Can you work these out from the model? Positions are in its coordinate system, mm. Face numbers are marked on the shaded views. Give positions to 0.01 mm unless a question says otherwise; leave off trailing zeros. Write each loop counter-clockwise with the first axis right and the second up, starting at its lowest first coordinate (ties: lowest second). Pieces come first, ordered by that corner, then holes. Notation, with made-up numbers: (-28, -14) -> (-12, -14) arc R5 ccw to (-12, -6) -> close; hole circle Ø11 at (-12, -0.5). An arc over 180 degrees is marked (long way). Answer as CSV lines item,"result". Start each with the question number.
1. I need wall thicknesses on line 1 (X direction, y = -26, z = 5); line 2 (Y direction, x = -15.5, z = 3.5); line 3 (X direction, y = -1, z = 5). Which ranges of each line are inside material? Lowest first, please. Write a range as [from, to].
2. If we section it at A-A on y = -14.5: Write out the boundary of the cut face in (x, z), plus the area to 3 significant figures.
3. If we section it at B-B on z = 2.25: Write out the boundary of the cut face in (x, y).
4. If we section it at C-C on y = 40.5: Write out the boundary of the cut face in (x, z), plus the area to 3 significant figures.
5. If we mould it in two halves opening along Z, with no side actions, what happens to the marked faces 1 and 2? For each: pulls with the +Z half, pulls with the -Z half, needs draft (parallel to the pull), parting line crosses it, or undercut.
6. I'm going to push a flat-ended pin straight in: P1, Ø6, axis at x = -62, y = 57, coming from the -Z side. Where does the tip first touch, or does it pass through?
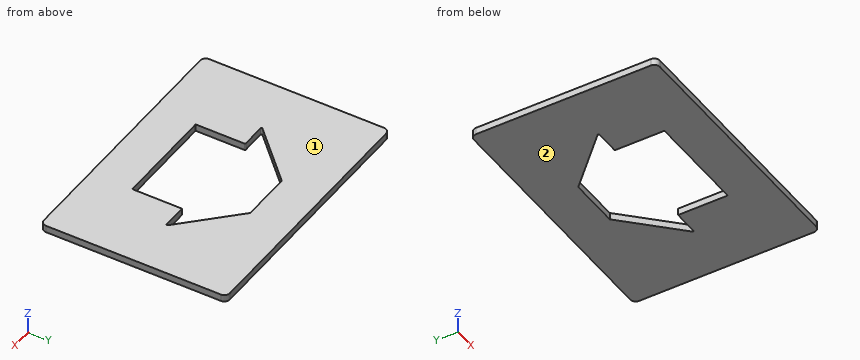
```python
from build123d import *

# Parameters (mm, degrees)
F0_W     = 238.125
F0_H     = 168.275
F1_DEPTH = 6.35
F3_DEPTH = 6.351
F5_DEPTH = 6.351
F6_R     = 5.08


with BuildPart() as f1:
    # F0 (on Top) → F1 (new body)
    with BuildSketch(Plane.XY):
        Rectangle(F0_W, F0_H)
    extrude(amount=F1_DEPTH)

    # F2 (on face) → F3 (cut, through all)
    with BuildSketch(Plane.XY.offset(6.35)):
        Polygon((22.479, 44.901281), (0, 44.901281), (-22.479, 44.901281), (-67.380281, 0), (-44.958, 0), (-44.958, -44.958), (0, -44.958), (44.958, -44.958), (44.958, 0), (67.380281, 0), align=None)
    extrude(amount=-F3_DEPTH, mode=Mode.SUBTRACT)

    # F4 (on face) → F5 (cut, through all)
    with BuildSketch(Plane.XY.offset(6.35)):
        with BuildLine():
            ThreePointArc((-22.678899, 46.171281), (-22.980224, 46.111343), (-23.235675, 45.940656))
            Line((-23.235675, 45.940656), (-69.102156, 0.074176))
            ThreePointArc((-69.102156, 0.074176), (-69.272843, -0.783925), (-68.54538, -1.27))
            Line((-68.54538, -1.27), (-47.0154, -1.27))
            ThreePointArc((-47.0154, -1.27), (-46.458624, -1.500624), (-46.228, -2.0574))
            Line((-46.228, -2.0574), (-46.228, -46.228))
            Line((-46.228, -46.228), (45.4406, -46.228))
            ThreePointArc((45.4406, -46.228), (45.997376, -45.997376), (46.228, -45.4406))
            Line((46.228, -45.4406), (46.228, -1.27))
            Line((46.228, -1.27), (68.54538, -1.27))
            ThreePointArc((68.54538, -1.27), (69.272843, -0.783925), (69.102156, 0.074176))
            Line((69.102156, 0.074176), (23.235675, 45.940656))
            ThreePointArc((23.235675, 45.940656), (22.980224, 46.111343), (22.678899, 46.171281))
            Line((22.678899, 46.171281), (-22.678899, 46.171281))
        make_face()
    extrude(amount=-F5_DEPTH, mode=Mode.SUBTRACT)

    # F6
    f6_edges = [f1.edges().sort_by_distance(p)[0] for p in [
        (119.0625, 84.1375, 3.175),
        (119.0625, -84.1375, 3.175),
        (-119.0625, -84.1375, 3.175),
        (-119.0625, 84.1375, 3.175),
    ]]
    fillet(f6_edges, radius=F6_R)


solid = f1.part
```
Computed values:
1,line 1,"x = [-119.06, -46.23], [46.23, 119.06]"
1,line 2,"y = [-84.14, -46.23], [46.17, 84.14]"
1,line 3,"x = [-119.06, -69.14], [69.14, 119.06]"
2,outline,"(-119.06, 0) -> (-46.23, 0) -> (-46.23, 6.35) -> (-119.06, 6.35) -> close; (46.23, 0) -> (119.06, 0) -> (119.06, 6.35) -> (46.23, 6.35) -> close"
2,area,"925 mm2"
3,outline,"(-119.06, -79.06) arc R5.08 ccw to (-113.98, -84.14) -> (113.98, -84.14) arc R5.08 ccw to (119.06, -79.06) -> (119.06, 79.06) arc R5.08 ccw to (113.98, 84.14) -> (-113.98, 84.14) arc R5.08 ccw to (-119.06, 79.06) -> close; hole (-69.1, 0.07) arc R0.79 ccw to (-68.55, -1.27) -> (-47.02, -1.27) arc R0.79 cw to (-46.23, -2.06) -> (-46.23, -46.23) -> (45.44, -46.23) arc R0.79 ccw to (46.23, -45.44) -> (46.23, -1.27) -> (68.55, -1.27) arc R0.79 ccw to (69.1, 0.07) -> (23.24, 45.94) arc R0.79 ccw to (22.68, 46.17) -> (-22.68, 46.17) arc R0.79 ccw to (-23.24, 45.94) -> close"
4,outline,"(-119.06, 0) -> (-28.68, 0) -> (-28.68, 6.35) -> (-119.06, 6.35) -> close; (28.68, 0) -> (119.06, 0) -> (119.06, 6.35) -> (28.68, 6.35) -> close"
4,area,"1,150 mm2"
5,face 1,"pulls with the +Z half"
5,face 2,"pulls with the -Z half"
6,P1,"stops at z = 0"
